Study the drawing (mm; zero at the part's minimum x, y, z) and answer. Round coordinates to 2 decimals unless told otherwise and drop trailing zeros. Order: outer loops, then holes, each group sorted by start corner. A loop starts at its lowest first (then second) coordinate and runs counter-clockwise, first axis right, second up. Notation, with made-up numbers: (64.25, -5) -> (85.25, -5) arc R8 cw to (85.25, 7) -> close; hole circle Ø6 at (31.5, -12.75). An arc over 180 degrees is marked (long way). Use one line per item in the form item = value.
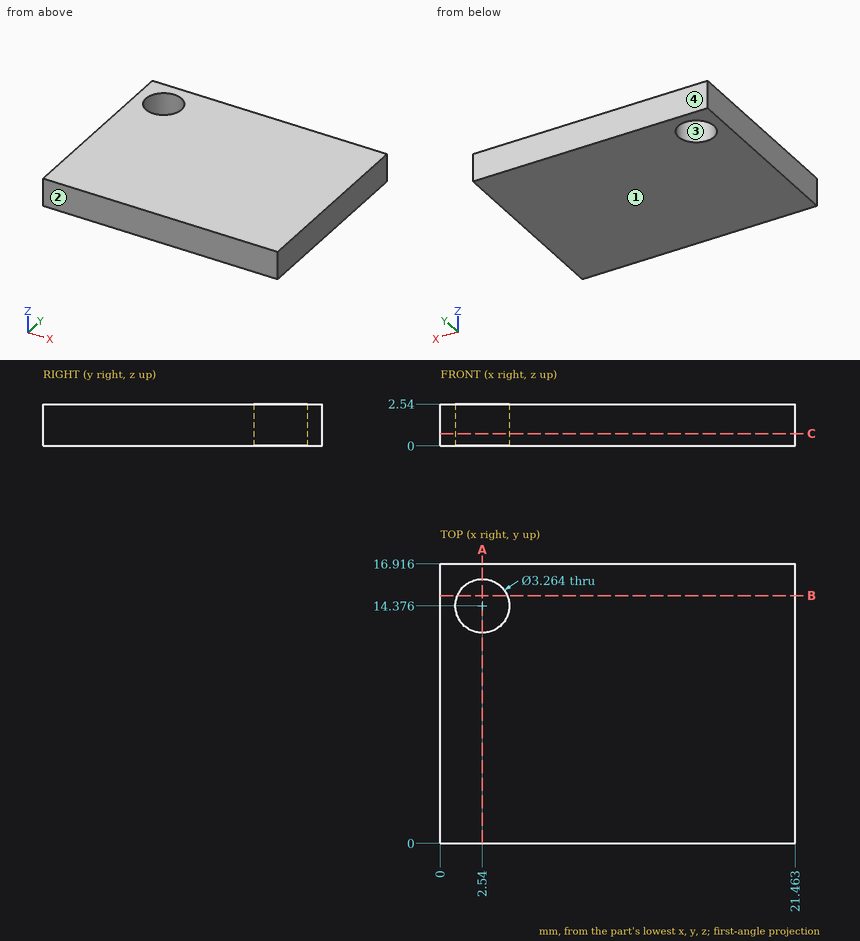
Item 1: The part is cut by section C-C, the plane z = 0.75. Give the vertices of the cut face in (x, y).
Findings:
outline = (0, 0) -> (21.46, 0) -> (21.46, 16.92) -> (0, 16.92) -> close; hole circle Ø3.26 at (2.54, 14.38)
Item 2: The part is cut by section B-B, the plane y = 15. Give the vertices of the cut face in (x, z).
Findings:
outline = (0, 0) -> (1.03, 0) -> (1.03, 2.54) -> (0, 2.54) -> close; (4.05, 0) -> (21.46, 0) -> (21.46, 2.54) -> (4.05, 2.54) -> close
Item 3: A flat-ended cylindrical pin translates along its axis: P1, Ø3, axis at x = 7, y = 12.5, coming from the -Z side. Find the tip coordinate at first contact, or state that the pin passes through.
Findings:
P1 = 0
Item 4: Determine the mould class of the marked faces 1, 2, 3 and 4 for opening direction Y: released by +Y, released by -Y, zero draft, split by the parting line, or undercut.
Findings:
face_1 = zero draft
face_2 = released by -Y
face_3 = undercut
face_4 = released by +Y
Item 5: The part is cut by section A-A, the plane x = 2.54. Give the vertices of the cut face in (y, z) (1 decimal).
Findings:
outline = (0, 0) -> (12.7, 0) -> (12.7, 2.5) -> (0, 2.5) -> close; (16, 0) -> (16.9, 0) -> (16.9, 2.5) -> (16, 2.5) -> close
Item 6: Consider line 1 along Y through (x, z) = (2.54, 0.75) (1 decimal); line 2 along X through (y, z) = (14.25, 1.5); line 3 along X through (y, z) = (13.5, 0.8) (1 decimal). Determine where each line is inside the solid, lowest interval first.
Findings:
line_1 = 0 to 12.7, 16 to 16.9
line_2 = 0 to 0.91, 4.17 to 21.46
line_3 = 0 to 1.2, 3.9 to 21.5
